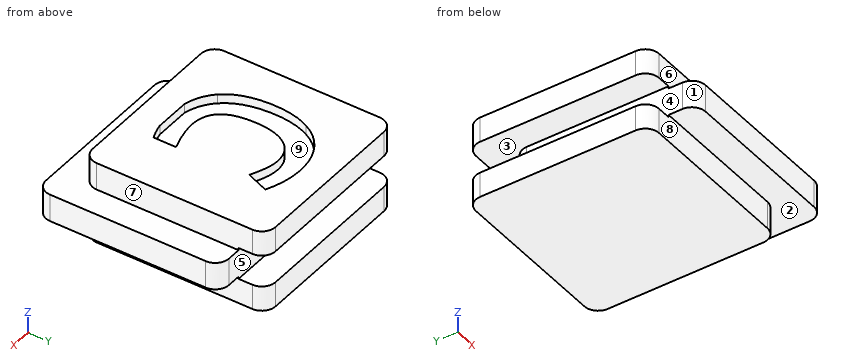
from build123d import *

# Parameters (mm, degrees)
F0_W     = 14
F0_H     = 3
F0_W_2   = 3
F1_DEPTH = 20
F2_DEPTH = 3
F3_W     = 3
F3_H     = 3
F4_DEPTH = 100
F5_W     = 3
F5_H     = 3.5
F6_DEPTH = 100
F7_R     = 1.5
F9_DEPTH = 1


with BuildPart() as f1:
    # F0 (on Front) → F1 (new body)
    with BuildSketch(Plane.XZ):
        Polygon((10, 1.5), (10, 4.5), (-10, 4.5), (-10, 1.5), (-7, 1.5), (7, 1.5), align=None)
        Rectangle(F0_W, F0_H)
        with Locations((11.5, 0)):
            Rectangle(F0_W_2, F0_H)
        with Locations((8.5, 0)):
            Rectangle(F0_W_2, F0_H)
        with Locations((-8.5, 0)):
            Rectangle(F0_W_2, F0_H)
        Polygon((10, -4.5), (10, -1.5), (7, -1.5), (-7, -1.5), (-10, -1.5), (-10, -4.5), align=None)
    extrude(amount=-F1_DEPTH)

    # F0 (on Front) → F2 (join)
    with BuildSketch(Plane.XZ):
        with Locations((-8.5, 0)):
            Rectangle(F0_W_2, F0_H)
        Rectangle(F0_W, F0_H)
        with Locations((8.5, 0)):
            Rectangle(F0_W_2, F0_H)
        with Locations((11.5, 0)):
            Rectangle(F0_W_2, F0_H)
    extrude(amount=F2_DEPTH)

    # F3 (on face) → F4 (cut)
    with BuildSketch(Plane.YZ.offset(13)):
        Polygon((23, -1.75), (23, 1.75), (17, 1.75), (17, 1.5), (20, 1.5), (20, -1.5), (17, -1.5), (17, -1.75), align=None)
        with Locations((18.5, 0)):
            Rectangle(F3_W, F3_H)
    extrude(amount=-F4_DEPTH, mode=Mode.SUBTRACT)

    # F5 (on face) → F6 (cut)
    with BuildSketch(Plane(origin=(0, 17, 0), x_dir=(-1, 0, 0), z_dir=(0, 1, 0))):
        with Locations((11.5, 0)):
            Rectangle(F5_W, F5_H)
        with Locations((8.5, 0)):
            Rectangle(F5_W, F5_H)
    extrude(amount=-F6_DEPTH, mode=Mode.SUBTRACT)

    # F7
    f7_edges = [f1.edges().sort_by_distance(p)[0] for p in [
        (-7, -3, 0),
        (13, -3, 0),
        (10, 0, 3),
        (10, 0, -3),
        (-10, 0, -3.125),
        (-10, 0, 3.125),
        (-7, 17, 0),
        (-10, 20, 3.125),
        (-10, 20, -3.125),
        (13, 17, 0),
        (10, 20, 3.125),
        (10, 20, -3.125),
    ]]
    fillet(f7_edges, radius=F7_R)

    # F8 (on face) → F9 (cut)
    with BuildSketch(Plane.XY.offset(4.5)):
        with BuildLine():
            Line((-1.6191336456, 3), (2.2633536651, 3))
            add(Edge.make_bspline(
                [(4.0033986182, 3.5225694444), (3.1800065383, 3.1782684858), (2.2633536651, 3)],
                knots=[0, 0, 0, 0.4822306436, 0.4822306436, 0.4822306436], degree=2))
            Line((4.0033986182, 3.5225694444), (4.0033986182, 5.9895833333))
            add(Edge.make_bspline(
                [(0.4639020904, 5.2604166667), (1.9252736182, 5.2604166667), (4.0033986182, 5.9895833333)],
                knots=[0, 0, 0, 1, 1, 1], degree=2))
            add(Edge.make_bspline(
                [(-3.0209069374, 9.9027777778), (-3.0209069374, 5.2604166667), (0.4639020904, 5.2604166667)],
                knots=[0, 0, 0, 1, 1, 1], degree=2))
            add(Edge.make_bspline(
                [(-2.109448604, 13.3815104167), (-3.0209069374, 12.1328125), (-3.0209069374, 9.9027777778)],
                knots=[0, 0, 0, 1, 1, 1], degree=2))
            add(Edge.make_bspline(
                [(0.4639020904, 14.6302083333), (-1.1979902707, 14.6302083333), (-2.109448604, 13.3815104167)],
                knots=[0, 0, 0, 1, 1, 1], degree=2))
            add(Edge.make_bspline(
                [(2.0103430626, 14.3552517361), (1.2234507015, 14.6302083333), (0.4639020904, 14.6302083333)],
                knots=[0, 0, 0, 1, 1, 1], degree=2))
            add(Edge.make_bspline(
                [(3.578051396, 13.7096354167), (2.7972354237, 14.0802951389), (2.0103430626, 14.3552517361)],
                knots=[0, 0, 0, 1, 1, 1], degree=2))
            Line((3.578051396, 13.7096354167), (4.5259680626, 16.1037326389))
            add(Edge.make_bspline(
                [(0.4639020904, 17.0789930556), (2.484301396, 17.0789930556), (4.5259680626, 16.1037326389)],
                knots=[0, 0, 0, 1, 1, 1], degree=2))
            add(Edge.make_bspline(
                [(-2.9966013818, 16.2115885417), (-1.5200388818, 17.0789930556), (0.4639020904, 17.0789930556)],
                knots=[0, 0, 0, 1, 1, 1], degree=2))
            add(Edge.make_bspline(
                [(-5.2615753401, 13.7157118056), (-4.4731638818, 15.3441840278), (-2.9966013818, 16.2115885417)],
                knots=[0, 0, 0, 1, 1, 1], degree=2))
            add(Edge.make_bspline(
                [(-6.0499867985, 9.9210069444), (-6.0499867985, 12.0872395833), (-5.2615753401, 13.7157118056)],
                knots=[0, 0, 0, 1, 1, 1], degree=2))
            add(Edge.make_bspline(
                [(-4.4458201318, 4.6467013889), (-6.0499867985, 6.4848090278), (-6.0499867985, 9.9210069444)],
                knots=[0, 0, 0, 1, 1, 1], degree=2))
            add(Edge.make_bspline(
                [(-1.6191336456, 3), (-3.3593104462, 3.4017423741), (-4.4458201318, 4.6467013889)],
                knots=[0.3226952609, 0.3226952609, 0.3226952609, 1, 1, 1], degree=2))
        make_face()
    extrude(amount=-F9_DEPTH, mode=Mode.SUBTRACT)


solid = f1.part
Build history of the part. All positions in model axes, mm. Face numbers are marked on the shaded views. A direction names the side the tool comes from. Coordinates: 2 decimals unless noted, no trailing zeros. Write each loop counter-clockwise with the first axis right and the second up, starting at its lowest first coordinate (ties: lowest second). Pieces come first, ordered by that corner, then holes. Notation, with made-up numbers: (-11, -7.75) -> (40, -7.75) arc R32 ccw to (40, 27.25) -> close; hole circle Ø11 at (51.25, -25.5). An arc over 180 degrees is marked (long way). Use CSV: the item, a comma, the result in double quotes. Start each with the question number.
Q1. Pull direction Z, two halves, no side cores. Call the marked faces 1, 2, 3 and 4: released by +Z, released by -Z, zero draft, split by the parting line, or undercut.
Q2. Cut at A-A, the plane x = -8. List the corners of the cut face in (y, z), then the cut area to 3 significant figures.
Q3. Drill centre lines: probe 1 along Z at (x, y) = (5, 18); probe 2 along Y at (x, z) = (9.5, -0.5); probe 3 along X at (y, z) = (2, 0). Where is each one in solid material? Low to high.
Q4. Cut at B-B, the plane z = 1. List the corners of the cut face in (x, y), then the cut area to 3 significant figures.
Q5. Flat gauge pins, fed straight in: pin 1 Ø3 at (y, z) = (-0.5, 3) entering from -X; pin 2 Ø1.5 at (y, z) = (7.5, -3) entering from +X; pin 3 Ø3.5 at (x, z) = (-3, -3.5) entering from -Y. Where does each tip first touch, or does it go through?
Q6. 3-axis set-ups, long thin cutter, end or side, ignore diameter. For the marked faces 5, 6, 7, 8 and 9: which of +Z, -Z, +X, -X, +Y, -Y reach the whole face in a straight line?
Checked values:
1,face 1,"zero draft"
1,face 2,"released by -Z"
1,face 3,"undercut"
1,face 4,"undercut"
2,outline,"(0, -4.5) -> (20, -4.5) -> (20, -1.75) -> (0, -1.75) -> close; (0, 1.75) -> (20, 1.75) -> (20, 4.5) -> (0, 4.5) -> close"
2,area,"110 mm²"
3,probe 1,"z = -4.5 to -1.75, 1.75 to 4.5"
3,probe 2,"y = -3 to 17"
3,probe 3,"x = -7 to 13"
4,outline,"(-7, -1.5) arc R1.5 ccw to (-5.5, -3) -> (11.5, -3) arc R1.5 ccw to (13, -1.5) -> (13, 15.5) arc R1.5 ccw to (11.5, 17) -> (-5.5, 17) arc R1.5 ccw to (-7, 15.5) -> close"
4,area,"398 mm²"
5,pin 1,"stops at x = -9.91"
5,pin 2,"stops at x = 10"
5,pin 3,"stops at y = 0"
6,face 5,"+X, -X, +Y"
6,face 6,"+Z, +X, -X, -Y"
6,face 7,"+Z, +X, +Y, -Y"
6,face 8,"-Z, +X, -X, -Y"
6,face 9,"+Z"
